from build123d import *

# Parameters (mm, degrees)
CYLINDER002_R           = 0.25
CYLINDER002_DEPTH       = 10
CYLINDER002_PITCH_ANGLE = 90
CYLINDER001_R           = 0.25
CYLINDER001_DEPTH       = 10
CYLINDER001_PITCH_ANGLE = 90
BOX_W                   = 6.5
BOX_H                   = 4.8
BOX_DEPTH               = 1


with BuildPart() as cylinder002:
    # Cylinder002 → Cylinder002 (new body)
    with BuildSketch(Plane.XY):
        Circle(CYLINDER002_R)
    extrude(amount=CYLINDER002_DEPTH)


with BuildPart() as cylinder002_1:
    # Cylinder002 pitch: moved
    add(cylinder002.part.rotate(Axis((0, 0, 0), (0, 1, 0)), CYLINDER002_PITCH_ANGLE))


with BuildPart() as cylinder002_2:
    # Cylinder002 placement: moved
    add(cylinder002_1.part.moved(Location((0, -2, -3.7))))


with BuildPart() as fusion002:
    # Cylinder001 → Cylinder001 (new body)
    with BuildSketch(Plane.XY):
        Circle(CYLINDER001_R)
    extrude(amount=CYLINDER001_DEPTH)


with BuildPart() as fusion002_1:
    # Cylinder001 pitch: moved
    add(fusion002.part.rotate(Axis((0, 0, 0), (0, 1, 0)), CYLINDER001_PITCH_ANGLE))


with BuildPart() as fusion002_2:
    # Cylinder001 placement: moved
    add(fusion002_1.part.moved(Location((-11, 2, -3.7))))

    # Fusion002: union Cylinder002
    add(cylinder002_2.part)


with BuildPart() as switch:
    # Box → Box (new body)
    with BuildSketch(Plane(origin=(-3.25, -2.4, -4.2), x_dir=(1, 0, 0), z_dir=(0, 0, 1))):
        with Locations((3.25, 2.4)):
            Rectangle(BOX_W, BOX_H)
    extrude(amount=BOX_DEPTH)

    # Fusion003: union Fusion002
    add(fusion002_2.part)


solid = switch.part
Verification items for the finished model (mm, model axes). Give positions to 0.01 mm unless a question says otherwise; leave off trailing zeros. Order: outer loops, then holes, each group sorted by start corner. A loop starts at its lowest first (then second) coordinate and runs counter-clockwise, first axis right, second up. Notation, with made-up numbers: M 57.5,66 L 114.5,66 A17 cw 114.5,74 Z; hole C 15,42.5 d9. An arc over 180 degrees is marked long. Answer as a JSON object with one key per item and string values. Group by question number.
1) Cross-section at D-D (y = 0.45). Enter the section's corners in (x, z), then the cut area to 3 significant figures.
2) Cross-section at C-C (y = -2). Enter the section's corners in (x, z), then the cut area to 4 significant figures.
3) Cross-section at B-B (y = 2). Enter the section's corners in (x, z).
4) Scan lines: line 1 along X through (y, z) = (-1.3, -4); line 2 along X through (y, z) = (1.85, -3.7); line 3 along Y through (x, z) = (-7.25, -3.5). Record each from-to range of solid material in increasing order. Write a range as [from, to].
5) Cross-section at A-A (z = -3.7). Enter the section's corners in (x, y).
Result sheet:
{
 "1": {"outline": "M -3.25,-4.2 L 3.25,-4.2 L 3.25,-3.2 L -3.25,-3.2 Z", "area": "6.50 mm2"},
 "2": {"outline": "M -3.25,-4.2 L 3.25,-4.2 L 3.25,-3.95 L 10,-3.95 L 10,-3.45 L 3.25,-3.45 L 3.25,-3.2 L -3.25,-3.2 Z", "area": "9.875 mm2"},
 "3": {"outline": "M -11,-3.95 L -3.25,-3.95 L -3.25,-4.2 L 3.25,-4.2 L 3.25,-3.2 L -3.25,-3.2 L -3.25,-3.45 L -11,-3.45 Z"},
 "4": {"line 1": "x = [-3.25, 3.25]", "line 2": "x = [-11, 3.25]", "line 3": "y = [1.85, 2.15]"},
 "5": {"outline": "M -11,1.75 L -3.25,1.75 L -3.25,-2.4 L 3.25,-2.4 L 3.25,-2.25 L 10,-2.25 L 10,-1.75 L 3.25,-1.75 L 3.25,2.4 L -3.25,2.4 L -3.25,2.25 L -11,2.25 Z"}
}
